Can you work these out from the drawing? Everything is in mm from the part's minimum corner. A direction names the side the tool comes from. Coordinates: 2 decimals unless noted, no trailing zeros. Loops run counter-clockwise (first coordinate to the right, second up) from the corner with the lowest first, then second, coordinate; pieces in that order, holes last. Notation, with made-up numbers: M 17.5,69.25 L 70.5,69.25 A15 cw 70.5,92.25 Z; hole C 31.5,34.5 d1. An arc over 180 degrees is marked long. Use CSV: the item, a comma, the result in double quotes. Start each with the question number.
Q1. If we mould it in two halves opening along Y, with no side actions, what happens to the marked faces 1, 2 and 3? For each: +Y half, -Y half, draft (parallel to the pull), parting line (faces both ways), or undercut.
Q2. If we section it at B-B (z = 1.95): Please give me the cut outline in (x, y), and give its area (3 significant figures).
Q3. Which directions (+Z, -Z, +X, -X, +Y, -Y) give clear straight access to the entire face, cutting with the end or side of a thin tool? Please do the marked faces 4 and 5.
Q4. If we section it at C-C (y = 13): Please give me the cut outline in (x, z).
Q5. Please list where these lines run through material, in increasing order: probe 1 along Y at (x, z) = (7.5, 2.75); probe 2 along X at (y, z) = (31, 0.8); probe 3 along X at (y, z) = (39, 2.2). Write a range as [from, to].
Q6. If we section it at D-D (x = 1.5): Please give me the cut outline in (y, z).
Q7. For pin 1 Ø3 at (x, y) = (6, 18.5) entering from -Z; pin 2 Ø3 at (y, z) = (28, 3.5) entering from +X, each with a flat end and sliding along its axis, tell me the tip position at first contact or that it passes through.
Q8. If we section it at A-A (x = 18.5): Please give me the cut outline in (y, z), and give its area (3 significant figures).
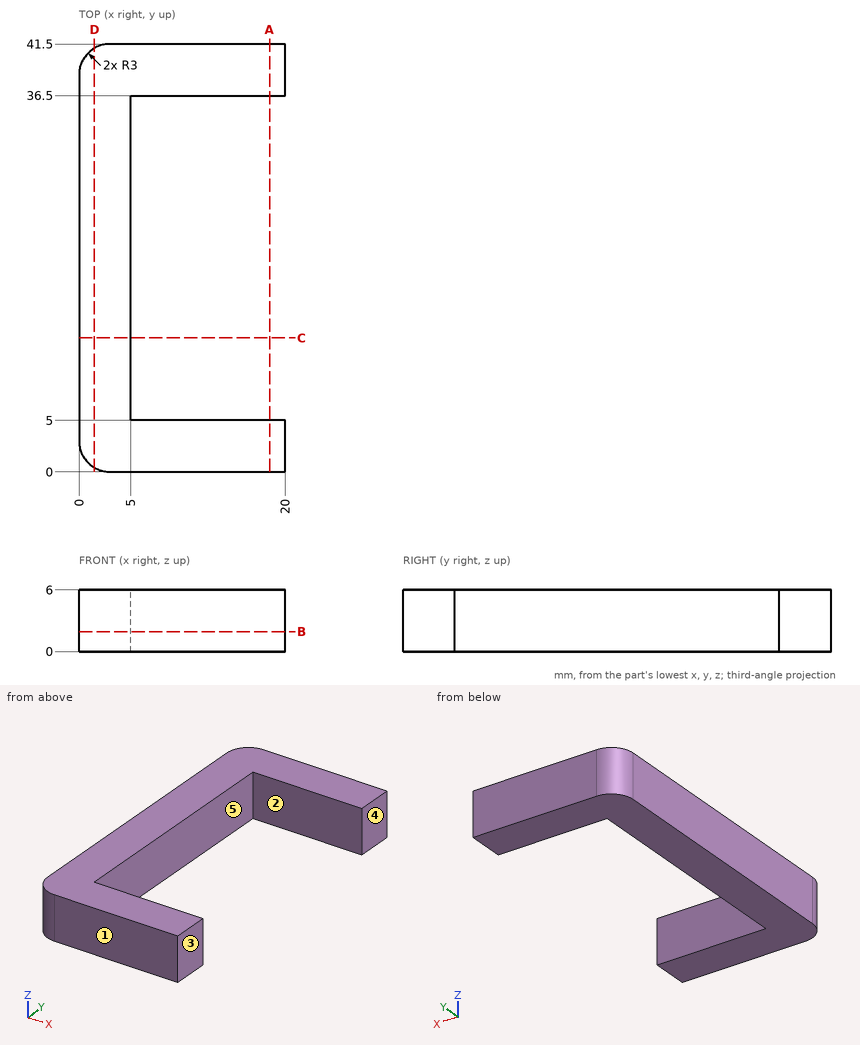
Results below:
1,face 1,"-Y half"
1,face 2,"undercut"
1,face 3,"draft"
2,outline,"M 0,3 A3 ccw 3,0 L 20,0 L 20,5 L 5,5 L 5,36.5 L 20,36.5 L 20,41.5 L 3,41.5 A3 ccw 0,38.5 Z"
2,area,"354 mm^2"
3,face 4,"+Z, -Z, +X, +Y, -Y"
3,face 5,"+Z, -Z, +X"
4,outline,"M 0,0 L 5,0 L 5,6 L 0,6 Z"
5,probe 1,"[0, 5], [36.5, 41.5]"
5,probe 2,"[0, 5]"
5,probe 3,"[0.04, 20]"
6,outline,"M 0.4,0 L 41.1,0 L 41.1,6 L 0.4,6 Z"
7,pin 1,"z = 0"
7,pin 2,"x = 5"
8,outline,"M 0,0 L 5,0 L 5,6 L 0,6 Z; M 36.5,0 L 41.5,0 L 41.5,6 L 36.5,6 Z"
8,area,"60.0 mm^2"
